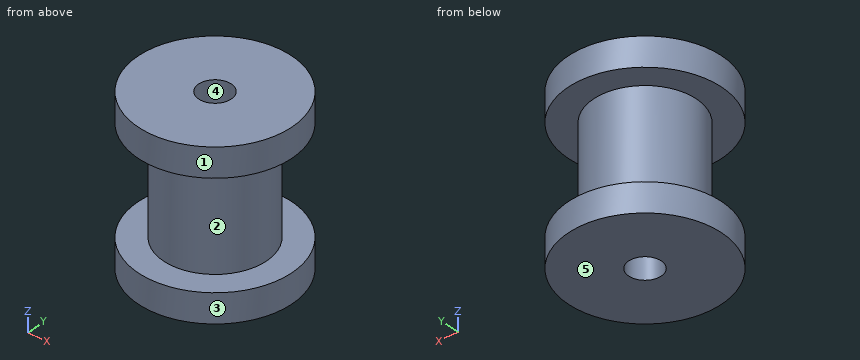
Autodesk Inventor part; units mm, degrees
ref_plane "Work Plane1" through (0, 0, -5.5) normal (0, 0, 1) x (1, 0, 0)
ref_plane "YZ Plane" through (0, 0, 0) normal (1, 0, 0) x (0, 1, 0)
ref_plane "XZ Plane" through (0, 0, 0) normal (0, 1, 0) x (-1, 0, 0)
sketch "Sketch1" plane through (0, 0, 0) normal (1, 0, 0) x (0, 1, 0)
  line L0 (0, 0) -> (-5.36, 0)
  line L1 (-5.36, 0) -> (-5.36, -11)
  line L2 (-5.36, -11) -> (0, -11)
  line L3 (0, -11) -> (0, 0)
  line L4 (0, -11) -> (-8, -11)
  line L5 (-8, -11) -> (-8, -14)
  line L6 (-8, -14) -> (0, -14)
  line L7 (0, -14) -> (0, -11)
  line L8 (0, 0) -> (-8, 0)
  line L9 (-8, 0) -> (-8, 3)
  line L10 (-8, 3) -> (0, 3)
  line L11 (0, 3) -> (0, 0)
  dimension "d0" = 5.36
  dimension "d1" = 11
  dimension "d10" = 8
  dimension "d11" = 3
  dimension "d12" = 8
  dimension "d13" = 3
revolve "Revolution1" add sketch "Sketch1" angle 360 about axis through (0, 0, -11) along (0, 0, 1)
sketch "Sketch3" plane through (0, 0, 3) normal (0, 0, 1) x (1, 0, 0)
  point P0 (0, 0)
  point P1 (0, 0)
hole "Hole2" at (0, 0, 3) direction (0, 0, -1) diameter 3.4 end through all
ref_plane "Work Plane1" through (0, 0, -5.5) normal (0, 0, 1) x (1, 0, 0)
properties part number "PuleyIdlerHolder" material "ABS Plastic"
Read the model definition and answer for the solid it produces. Units are mm, in the model's axes. Face numbers are marked on the shaded views. A direction names the side the tool comes from. Give positions to 0.01 mm unless a question says otherwise; leave off trailing zeros. Write each loop counter-clockwise with the first axis right and the second up, starting at its lowest first coordinate (ties: lowest second). Pieces come first, ordered by that corner, then holes. Notation, with made-up numbers: (32, 40) - (39, 40) arc R26 cw to (39, 70) - close; hole circle Ø1 at (-11.5, 25). An arc over 180 degrees is marked (long way). Answer in a Markdown table with one row per item. Add a question column.
Item 1: Flat-ended cylindrical pins translate along their axes: P1, Ø1.5, axis at x = 4, z = -4.5, coming from the +Y side; P2, Ø4, axis at y = -5.5, z = -12, coming from the +X side; P3, Ø1.5, axis at x = -1, z = -7.5, coming from the +Y side. Find the tip coordinate at first contact, or state that the pin passes through.
Item 2: A tool of negligible diameter and unlimited length cuts with its end or side. For the marked faces 1 and 2, from which of +Z, -Z, +X, -X, +Y, -Y can it reach the whole face along a straight path? Write none if from no direction.
Item 3: Find the intervals of material crossed by L1, parallel to X at y = 0, z = -6.75; L2, parallel to Z at x = 5.75, y = -1.25; L3, parallel to X at y = 1.5, z = -1, in increasing order.
Item 4: Determine the mould class of the marked faces 3, 4 and 5 for opening direction Y: pulls with the +Y half, pulls with the -Y half, needs draft (parallel to the pull), parting line crosses it, or undercut.
Item 5: Section C-C, the plane z = -7.75 is taken. Write down the section's boundary in (x, y).
Item 6: Section A-A, the plane x = 0 is taken. Write down the section's boundary in (y, z), and give its area (3 significant figures).
Item 7: Section D-D, the plane y = 4.5 is taken. Write down the section's boundary in (x, z).
Recorded:
| question | item | result |
|---|---|---|
| 1 | P1 | stops at y = 4.26 |
| 1 | P2 | stops at x = 7.19 |
| 1 | P3 | stops at y = 5.35 |
| 2 | face 1 | +Z, -Z |
| 2 | face 2 | none |
| 3 | L1 | x = -5.36 to -1.7, 1.7 to 5.36 |
| 3 | L2 | z = -14 to -11, 0 to 3 |
| 3 | L3 | x = -5.15 to -0.8, 0.8 to 5.15 |
| 4 | face 3 | parting line crosses it |
| 4 | face 4 | undercut |
| 4 | face 5 | needs draft |
| 5 | outline | circle Ø10.72 at (0, 0); hole circle Ø3.4 at (0, 0) |
| 6 | outline | (-8, -14) - (-1.7, -14) - (-1.7, 3) - (-8, 3) - (-8, 0) - (-5.36, 0) - (-5.36, -11) - (-8, -11) - close; (1.7, -14) - (8, -14) - (8, -11) - (5.36, -11) - (5.36, 0) - (8, 0) - (8, 3) - (1.7, 3) - close |
| 6 | area | 156 mm2 |
| 7 | outline | (-6.61, -14) - (6.61, -14) - (6.61, -11) - (2.91, -11) - (2.91, 0) - (6.61, 0) - (6.61, 3) - (-6.61, 3) - (-6.61, 0) - (-2.91, 0) - (-2.91, -11) - (-6.61, -11) - close |
